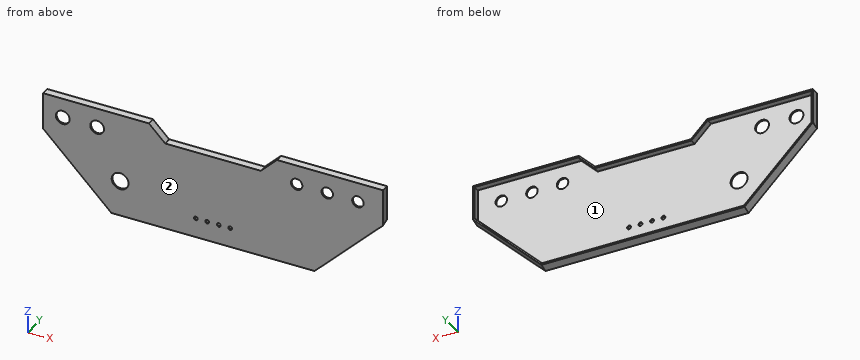
```python
from build123d import *

# Parameters (mm, degrees)
SHELL1_T           = -2
SKETCH4_R          = 2.5
SKETCH4_R_2        = 7.5
SKETCH4_R_3        = 9
SKETCH4_R_4        = 11
CUT_EXTRUDE1_DEPTH = 10


with BuildPart() as part:
    # Sketch1 → Loft2 section 0
    with BuildSketch(Plane(origin=(0, 0, 0), x_dir=(1, 0, 0), z_dir=(0, 1, 0))):
        Polygon((-132.627416996, -6), (132.627416996, -6), (221.999999995, -95.372582999), (221.999999995, -144), (83.69848481, -144), (62.485281374, -122.786796564), (-62.485281374, -122.786796564), (-83.69848481, -144), (-221.999999995, -144), (-221.999999995, -95.372582999), align=None)
    # Sketch2 → Loft2 section 1
    with BuildSketch(Plane(origin=(0, 10, 0), x_dir=(1, 0, 0), z_dir=(0, 1, 0))):
        Polygon((-83.698484794, -144), (-62.485281361, -122.786796562), (62.485281387, -122.786796547), (83.69848481, -143.999999995), (222.00000001, -143.999999995), (222.00000001, -98.149280245), (132.627417005, -8.77669724), (-132.627416995, -8.77669724), (-221.999999995, -98.14928025), (-221.999999995, -144), align=None)
    loft()

    # Shell1
    shell1_openings = [part.faces().sort_by_distance(p)[0] for p in [
        (8e-09, 10, 103.542554807),
    ]]
    offset(amount=SHELL1_T, openings=shell1_openings, kind=Kind.INTERSECTION)

    # Sketch4 → Cut-Extrude1 (cut)
    with BuildSketch(Plane.XZ):
        with Locations((22.5, 31.74)):
            Circle(SKETCH4_R)
        with Locations((7.5, 31.74)):
            Circle(SKETCH4_R)
        with Locations((-7.5, 31.74)):
            Circle(SKETCH4_R)
        with Locations((-22.5, 31.74)):
            Circle(SKETCH4_R)
        with Locations((189.259999995, 118.26)):
            Circle(SKETCH4_R_2)
        with Locations((149.259999995, 118.26)):
            Circle(SKETCH4_R_2)
        with Locations((109.259999995, 118.26)):
            Circle(SKETCH4_R_2)
        with Locations((-151.259999995, 118.26)):
            Circle(SKETCH4_R_3)
        with Locations((-196.259999995, 118.26)):
            Circle(SKETCH4_R_3)
        with Locations((-121.259999995, 53.26)):
            Circle(SKETCH4_R_4)
    extrude(amount=-CUT_EXTRUDE1_DEPTH, mode=Mode.SUBTRACT)


solid = part.part
```
Model file for the job. Use its own axes, mm. Face numbers are marked on the shaded views. Coordinates: 2 decimals unless noted, no trailing zeros. Return JSON: item names as keys, results as strings.
Item 1: Wall check: line 1 along Y through (x, z) = (-28.5, 27); line 2 along Z through (x, y) = (-151.26, 1.4); line 3 along X through (y, z) = (5.5, 109). Give the ranges that are in metal, low to high. Write a range as from..to.
Model answer:
{"line 1": "y = 0..2", "line 2": "z = 25.02..109.26, 127.26..144", "line 3": "x = -222..-220, 220..222"}
Item 2: Mould opens along X. For the marked faces 1 and 2 say: pulls with the +X half, pulls with the -X half, needs draft (parallel to the pull), parting line crosses it, or undercut.
Model answer:
{"face 1": "undercut", "face 2": "needs draft"}
Item 3: Pin check, flat tips, straight feed: P1, Ø24, axis at x = 109.26, z = 118.26, coming from the +Y side; P2, Ø4, axis at x = -174.5, y = 4.5, coming from the -Z side; P3, Ø2, axis at x = 54.5, y = 6.5, coming from the +Z side; P4, Ø13.5, axis at x = 189.26, z = 118.26, coming from the +Y side. Stop position of each tip, or through.
Model answer:
{"P1": "stops at y = 2", "P2": "stops at z = 47.05", "P3": "stops at z = 122.79", "P4": "passes through"}
